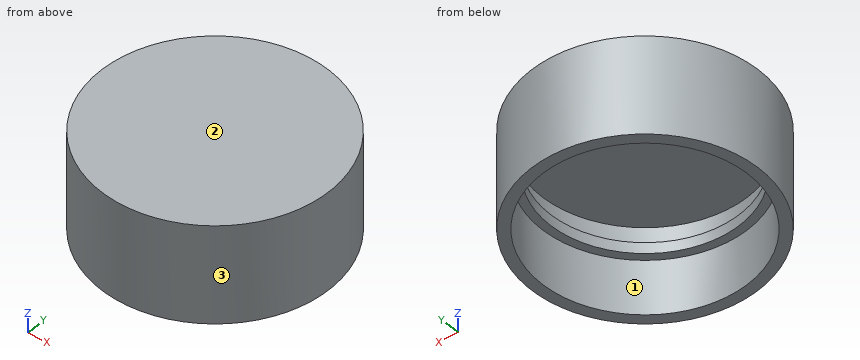
from build123d import *


with BuildPart() as part:
    # Skizze1 → Rotation2 (revolve)
    with BuildSketch(Plane(origin=(0, 0, 0), x_dir=(1, 0, 0), z_dir=(0, 1, 0)), mode=Mode.PRIVATE) as rotation2_sk:
        Polygon((0.00340061, -8.034840547), (0.00340061, -10.034840547), (20.90540061, -10.034840547), (20.90540061, 7.965159453), (18.90540061, 7.965159453), (18.90540061, -2.034840547), (17.40540061, -2.034840547), (17.40540061, -4.034840547), (18.90540061, -4.034840547), (18.90540061, -8.034840547), align=None)
    revolve(rotation2_sk.sketch.rotate(Axis((0.00340061, 0, 8.034840547), (0, 0, 1)), 180), axis=Axis((0.00340061, 0, 8.034840547), (0, 0, 1)))


solid = part.part
Build history of the part. All positions in model axes, mm. Face numbers are marked on the shaded views. Give positions to 0.01 mm unless a question says otherwise; leave off trailing zeros. Order: outer loops, then holes, each group sorted by start corner. A loop starts at its lowest first (then second) coordinate and runs counter-clockwise, first axis right, second up. Notation, with made-up numbers: M 25,-22 L 67,-22 A37 ccw 67,16 Z; hole C 27.5,26.25 d4. An arc over 180 degrees is marked long. Put each result on its own line as item: value.
Item 1: Cut at C-C on y = 0. Write the cut outline in (x, z), then the cut area to 3 significant figures.
Results are:
outline: M -20.9,-7.97 L -18.9,-7.97 L -18.9,2.03 L -17.4,2.03 L -17.4,4.03 L -18.9,4.03 L -18.9,8.03 L 18.91,8.03 L 18.91,4.03 L 17.41,4.03 L 17.41,2.03 L 18.91,2.03 L 18.91,-7.97 L 20.91,-7.97 L 20.91,10.03 L -20.9,10.03 Z
area: 154 mm2
Item 2: Wall check: probe 1 along Y at (x, z) = (-0.5, 0.5); probe 2 along Z at (x, y) = (-12, -10.5); probe 3 along X at (y, z) = (12, 0.75). Give the ranges that are in metal, low to high.
Results are:
probe 1: -20.9 to -18.9, 18.9 to 20.9
probe 2: 8.03 to 10.03
probe 3: -17.11 to -14.6, 14.61 to 17.12
Item 3: Drop flat-ended pins along their axis: pin 1 Ø8 at (y, z) = (9.5, 4) entering from +X; pin 2 Ø5 at (y, z) = (11.5, 5) entering from +X; pin 3 Ø1 at (y, z) = (-12.5, 6) entering from -X. Give the stop position or say it passes through.
Results are:
pin 1: x = 20.17
pin 2: x = 18.87
pin 3: x = -17.11
Item 4: Cut at D-D on x = 3. Write the cut outline in (y, z).
Results are:
outline: M -20.69,-7.97 L -18.66,-7.97 L -18.66,2.03 L -17.14,2.03 L -17.14,4.03 L -18.66,4.03 L -18.66,8.03 L 18.66,8.03 L 18.66,4.03 L 17.14,4.03 L 17.14,2.03 L 18.66,2.03 L 18.66,-7.97 L 20.69,-7.97 L 20.69,10.03 L -20.69,10.03 Z
Item 5: Cut at A-A on x = -18. Write the cut outline in (y, z).
Results are:
outline: M -10.62,-7.97 L -5.76,-7.97 L -5.76,2.03 L 5.76,2.03 L 5.76,-7.97 L 10.62,-7.97 L 10.62,10.03 L -10.62,10.03 Z; hole M -5.76,4.03 L 5.76,4.03 L 5.76,8.03 L -5.76,8.03 Z
Item 6: Pull direction Y, two halves, no side cores. Call the marked faces 1, 2 and 3: +Y half, -Y half, draft (parallel to the pull), parting line (faces both ways), or undercut.
Results are:
face 1: undercut
face 2: draft
face 3: parting line
Item 7: Cut at B-B on z = 3.5. Write the cut outline in (x, y).
Results are:
outline: C 0,0 d41.8; hole C 0,0 d34.8
